Input: dimensioned drawing with shaded views. Units: mm. Origin: part minimum x, y, z. A direction names the side the tool comes from. Coordinates: 2 decimals unless noted, no trailing zeros. Write each loop counter-clockwise with the first axis right and the second up, starting at its lowest first coordinate (ties: lowest second). Pieces come first, ordered by that corner, then holes. Notation, with made-up numbers: (10.25, 60) -> (45.25, 60) arc R32 cw to (45.25, 96) -> close; hole circle Ø3 at (-6, 34.5). An arc over 180 degrees is marked (long way). One line per item, written item: value. Start each with the question number.
1. Access query for the marked faces 1 and 2. Directions: +Z, -Z, +X, -X, +Y, -Y. A direction counts if a zero-diameter tool reaches every point of the face in a straight line with its end or side. Return the directions, or none.
2. First-contact query: P1, Ø5, axis at x = 20.5, y = 13, coming from the -Z side; P2, Ø2, axis at x = 5, z = 5, coming from the -Y side; P3, Ø6, axis at y = 2.5, z = 13, coming from the -X side; P4, Ø8, axis at x = 25, z = 9, coming from the +Y side. Flat tips, straight axial feed; report the tip coordinate or a pass-through.
3. Section query C-C, the plane x = 34. Output: boundary loops of the cut face in (y, z).
4. Section query A-A, the plane z = 8. Output: boundary loops of the cut face in (x, y), and give its area (4 significant figures).
5. Line query: line 1 (X direction, y = 9, z = 1.5); line 2 (Z direction, x = 32.5, y = 10.75); line 3 (Z direction, x = 22, y = 10.25). Output: solid intervals per line, ascending.
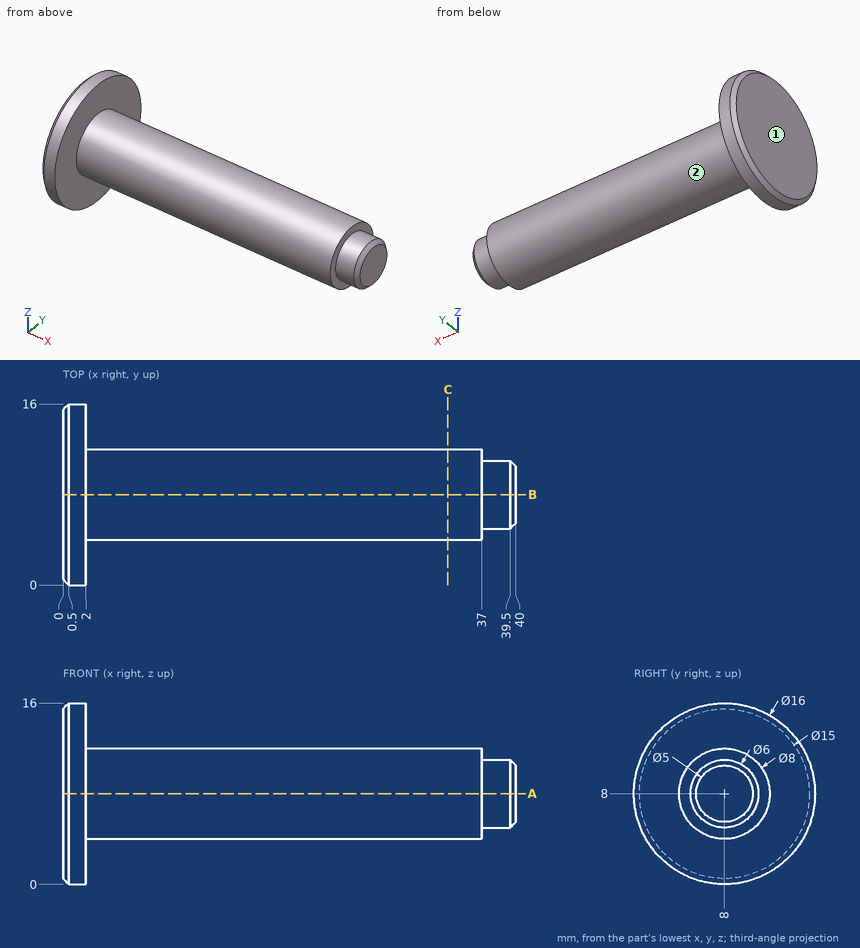
Computed values:
1. face 1: +Z, -Z, -X, +Y, -Y
1. face 2: +X
2. P1: stops at z = 4.88
2. P2: stops at y = 4.54
2. P3: stops at x = 0
2. P4: stops at y = 12
3. outline: circle Ø8 at (8, 8)
4. outline: (0, 0.5) -> (0.5, 0) -> (2, 0) -> (2, 4) -> (37, 4) -> (37, 5) -> (39.5, 5) -> (40, 5.5) -> (40, 10.5) -> (39.5, 11) -> (37, 11) -> (37, 12) -> (2, 12) -> (2, 16) -> (0.5, 16) -> (0, 15.5) -> close
4. area: 329.5 mm²
5. line 1: x = 0 to 2
5. line 2: z = 5.1 to 10.9
5. line 3: z = 4.69 to 11.31
